Source: CAD feature listing. Evaluate the final solid. Frame: model axes, mm. A direction names the side the tool comes from. Give positions to 0.01 mm unless a question says otherwise; leave off trailing zeros. Write each loop counter-clockwise with the first axis right and the second up, starting at its lowest first coordinate (ties: lowest second). Pieces come first, ordered by that corner, then holes. Notation, with made-up numbers: M 48,88.5 L 104,88.5 A18 cw 104,92.5 Z; hole C 6.25,6.25 d5. An arc over 180 degrees is marked long. Answer as a JSON object with one key per item and string values. Group by question number.
```python
from build123d import *

# Parameters (mm, degrees)
BOSS_EXTRUDE1_DEPTH = 50
BOSS_EXTRUDE2_DEPTH = 2
BOSS_EXTRUDE3_DEPTH = 2
SKETCH4_R           = 11
SKETCH4_R_2         = 1.75
CUT_EXTRUDE1_DEPTH  = 5
CUT_EXTRUDE2_DEPTH  = 5
CHAMFER1_SIZE       = 5


with BuildPart() as part:
    # Sketch1 → Boss-Extrude1 (new body)
    with BuildSketch(Plane(origin=(0, 0, 0), x_dir=(0, 0, -1), z_dir=(1, 0, 0))):
        with BuildLine():
            Line((0, 51), (0, 4))
            ThreePointArc((0, 4), (1.171572875, 1.171572875), (4, 0))
            Line((4, 0), (53, 0))
            Line((53, 0), (53, 2))
            Line((53, 2), (4, 2))
            ThreePointArc((4, 2), (2.585786438, 2.585786438), (2, 4))
            Line((2, 4), (2, 51))
            Line((2, 51), (0, 51))
        make_face()
    extrude(amount=-BOSS_EXTRUDE1_DEPTH)

    # Sketch2 → Boss-Extrude2 (add)
    with BuildSketch(Plane(origin=(0, 0, 0), x_dir=(0, 0, -1), z_dir=(1, 0, 0))):
        Polygon((2, 20), (13, 2), (5, 2), (2, 5), align=None)
    extrude(amount=-BOSS_EXTRUDE2_DEPTH)

    # Sketch3 → Boss-Extrude3 (add)
    with BuildSketch(Plane.ZY.offset(50)):
        Polygon((-2, 20), (-13, 2), (-5, 2), (-2, 5), align=None)
    extrude(amount=-BOSS_EXTRUDE3_DEPTH)

    # Sketch4 → Cut-Extrude1 (cut)
    with BuildSketch(Plane.XY):
        with Locations((-25, 30)):
            Circle(SKETCH4_R)
        with Locations((-9.5, 45.5)):
            Circle(SKETCH4_R_2)
        with Locations((-40.5, 45.5)):
            Circle(SKETCH4_R_2)
        with Locations((-40.5, 14.5)):
            Circle(SKETCH4_R_2)
        with Locations((-9.5, 14.5)):
            Circle(SKETCH4_R_2)
    extrude(amount=-CUT_EXTRUDE1_DEPTH, mode=Mode.SUBTRACT)

    # Sketch5 → Cut-Extrude2 (cut)
    with BuildSketch(Plane.XZ):
        with BuildLine():
            Line((-7.9, -42), (-7.9, -12))
            ThreePointArc((-7.9, -12), (-10, -9.9), (-12.1, -12))
            Line((-12.1, -12), (-12.1, -42))
            ThreePointArc((-12.1, -42), (-10, -44.1), (-7.9, -42))
        make_face()
        with BuildLine():
            Line((-37.9, -42), (-37.9, -12))
            ThreePointArc((-37.9, -12), (-40, -9.9), (-42.1, -12))
            Line((-42.1, -12), (-42.1, -42))
            ThreePointArc((-42.1, -42), (-40, -44.1), (-37.9, -42))
        make_face()
    extrude(amount=-CUT_EXTRUDE2_DEPTH, mode=Mode.SUBTRACT)

    # Chamfer1
    chamfer1_edges = [part.edges().sort_by_distance(p)[0] for p in [
        (0, 51, -1),
        (-50, 1, -53),
        (-50, 51, -1),
        (0, 1, -53),
    ]]
    chamfer(chamfer1_edges, length=CHAMFER1_SIZE)


solid = part.part
```
(1) Section C-C, the plane y = 30. Return loops of the section in (x, z).
(2) Section D-D, the plane x = -9.5. Return loops of the section in (y, z).
(3) Pull-direction query (X, two-part tool) for faces 1 (the flat face through (-47, 1, -51)), 2 (the cylindrical face through (-24.65, 1.203, -1.141)), 3 (the cylindrical face through (-39.69, 43.95, -0.99)); classes: pulls with the +X half, pulls with the -X half, needs draft (parallel to the pull), parting line crosses it, or undercut.
(4) Ray query, L1, parallel to Y at x = -40.5, z = -0.7; L2, parallel to Y at x = -9.5, z = -0.65; L3, parallel to Y at x = -26, z = -20.5. Return the intervals inside material, ascending. Write a range as [from, to].
(5) Section B-B, the plane z = -20. Return loops of the section in (x, y), plus the area to 3 significant figures.
(6) Section A-A, the plane x = -25. Return loops of the section in (y, z).
(7) Access query for faces 4 (the flat face through (-48, 48, -1)), 5 (the flat face through (-2, 7, -5)), 6 (the flat face through (-42.1, 1, -27)). Directions: +Z, -Z, +X, -X, +Y, -Y. A direction counts if a zero-diameter tool reaches every point of the face in a straight line with its end or side. Return the directions, or none.
(8) Contact query for flat-ended pins moving along their axis: pin 1 Ø12 at (x, z) = (-20.5, -30.5) entering from +Y; pin 2 Ø1.5 at (x, y) = (-44.5, 6) entering from -Z. Output: stop coordinate, or through.
Reported:
{
 "1": {"outline": "M -50,-2 L -36,-2 L -36,0 L -50,0 Z; M -14,-2 L 0,-2 L 0,0 L -14,0 Z"},
 "2": {"outline": "M 0,-53 L 2,-53 L 2,-44.04 L 0,-44.04 Z; M 0,-9.96 L 2,-9.96 L 2,-4 A2 cw 4,-2 L 12.75,-2 L 12.75,0 L 4,0 A4 ccw 0,-4 Z; M 16.25,-2 L 43.75,-2 L 43.75,0 L 16.25,0 Z; M 47.25,-2 L 51,-2 L 51,0 L 47.25,0 Z"},
 "3": {"face 1": "pulls with the -X half", "face 2": "needs draft", "face 3": "undercut"},
 "4": {"L1": "y = [1.74, 12.75], [16.25, 43.75], [47.25, 51]", "L2": "y = [1.81, 12.75], [16.25, 43.75], [47.25, 51]", "L3": "y = [0, 2]"},
 "5": {"outline": "M -50,0 L -42.1,0 L -42.1,2 L -50,2 Z; M -37.9,0 L -12.1,0 L -12.1,2 L -37.9,2 Z; M -7.9,0 L 0,0 L 0,2 L -7.9,2 Z", "area": "83.2 mm2"},
 "6": {"outline": "M 0,-53 L 2,-53 L 2,-4 A2 cw 4,-2 L 19,-2 L 19,0 L 4,0 A4 ccw 0,-4 Z; M 41,-2 L 51,-2 L 51,0 L 41,0 Z"},
 "7": {"face 4": "+Z, -Z, -X, +Y", "face 5": "-Z, +Y", "face 6": "+Y, -Y"},
 "8": {"pin 1": "stops at y = 2", "pin 2": "stops at z = -2"}
}
